```python
from build123d import *

# Parameters (mm, degrees)
SKETCH_1_R               = 15
SKETCH_1_R_2             = 1.25
EXTRUDE_2_DEPTH          = 5
SKETCH_3_R               = 5
EXTRUDE_4_DEPTH          = 1
SKETCH_4_R               = 3
CUT_EXTRUDE_1_DEPTH      = 5.5
CUT_EXTRUDE_2_DEPTH      = 78
CUT_EXTRUDE_2_DEPTH_BACK = 5.5
SKETCH_5_R               = 1.5


with BuildPart() as part:
    # ｽｹｯﾁ1 → ﾎﾞｽ - 押し出し2 (new body)
    with BuildSketch(Plane(origin=(0, 0, 0), x_dir=(0, 0, -1), z_dir=(1, 0, 0))):
        with Locations((27.213776389, 17.709467549)):
            Circle(SKETCH_1_R)
        with Locations((27.213776389, 29.709467549)):
            Circle(SKETCH_1_R_2, mode=Mode.SUBTRACT)
        with Locations((35.699057763, 26.194748924)):
            Circle(SKETCH_1_R_2, mode=Mode.SUBTRACT)
        with Locations((18.728495014, 26.194748924)):
            Circle(SKETCH_1_R_2, mode=Mode.SUBTRACT)
        with Locations((15.213776389, 17.709467549)):
            Circle(SKETCH_1_R_2, mode=Mode.SUBTRACT)
        with Locations((35.699057763, 9.224186175)):
            Circle(SKETCH_1_R_2, mode=Mode.SUBTRACT)
        with Locations((39.213776389, 17.709467549)):
            Circle(SKETCH_1_R_2, mode=Mode.SUBTRACT)
        with Locations((18.728495014, 9.224186175)):
            Circle(SKETCH_1_R_2, mode=Mode.SUBTRACT)
        with Locations((27.213776389, 5.709467549)):
            Circle(SKETCH_1_R_2, mode=Mode.SUBTRACT)
    extrude(amount=EXTRUDE_2_DEPTH)

    # ｽｹｯﾁ3 → ﾎﾞｽ - 押し出し4 (add)
    with BuildSketch(Plane(origin=(0, 0, 0), x_dir=(0, 0, -1), z_dir=(1, 0, 0))):
        with Locations((27.213776389, 17.709467549)):
            Circle(SKETCH_3_R)
    extrude(amount=-EXTRUDE_4_DEPTH)

    # ｽｹｯﾁ4 → ｶｯﾄ - 押し出し1 (cut)
    with BuildSketch(Plane(origin=(5, 0, 0), x_dir=(0, 0, -1), z_dir=(1, 0, 0))):
        with Locations((27.213776389, 17.709467549)):
            Circle(SKETCH_4_R)
    extrude(amount=-CUT_EXTRUDE_1_DEPTH, mode=Mode.SUBTRACT)

    # ｽｹｯﾁ5 → ｶｯﾄ - 押し出し2 (cut, two sides: drawn at the far end of the back side and taken through both)
    with BuildSketch(Plane.ZY.offset(-CUT_EXTRUDE_2_DEPTH_BACK)):
        with Locations(Location((-27.213776389, 17.709467549, 0), (0, 0, 180))):
            Circle(SKETCH_5_R)
    extrude(amount=CUT_EXTRUDE_2_DEPTH + CUT_EXTRUDE_2_DEPTH_BACK, mode=Mode.SUBTRACT)


solid = part.part
```
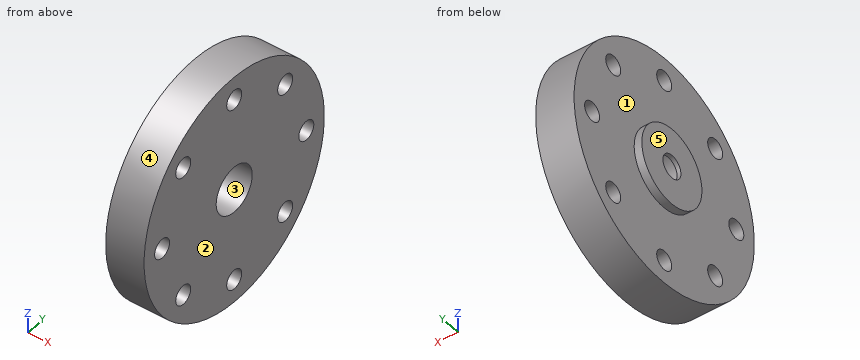
Could you check a few things on this model? Use its own coordinates, in mm. Face numbers are marked on the shaded views. A direction names the side the tool comes from. Round coordinates to 2 decimals unless told otherwise and drop trailing zeros. Loops run counter-clockwise (first coordinate to the right, second up) from the corner with the lowest first, then second, coordinate; pieces in that order, holes last. Notation, with made-up numbers: (44, -29.75) - (61, -29.75) arc R27 ccw to (61, -12.75) - close; hole circle Ø1 at (-30, 45.25). An arc over 180 degrees is marked (long way). Answer in a Markdown table with one row per item. Add a question column.
(1) I need wall thicknesses on line 1 along Y through (x, z) = (2.95, -19); line 2 along Y through (x, z) = (3.3, -27.5); line 3 along X through (y, z) = (10, -34). Which ranges of each line are inside material? Lowest first, please.
(2) If we section it at A-A (z = -18.5): Please give me the cut outline in (x, y).
(3) If we mould it in two halves opening along Y, with no side actions, what happens to the marked faces 3, 4 and 5? For each: pulls with the +Y half, pulls with the -Y half, needs draft (parallel to the pull), parting line crosses it, or undercut.
(4) If we section it at B-B (y = 27): Please give me the cut outline in (x, z), plus the area to 3 significant figures.
(5) If we section it at C-C (z = -28): Please give me the cut outline in (x, y).
(6) If we section it at D-D (y = 30.5): Please give me the cut outline in (x, z).
(7) I'm going to push flat-ended pins straight in: pin 1 (1 mm diameter, centred on x = 1.5, z = -18.5, fed in from +Y); pin 2 (2 mm diameter, centred on x = 2.5, z = -29.5, fed in from +Y); pin 3 (5 mm diameter, centred on y = 9.5, z = -23, fed in from -X). Where does each tip first touch, or does it pass through?
(8) For the marked faces 1 and 2, which set-ups out of +Z, -Z, +X, -X, +Y, -Y let a thin tool reach every point of the face, with its end or its side?
Model answer:
| question | item | result |
|---|---|---|
| 1 | line 1 | y = 5.16 to 8, 10.44 to 24.97, 27.41 to 30.26 |
| 1 | line 2 | y = 2.71 to 4.49, 6.93 to 14.72, 20.7 to 28.49, 30.93 to 32.71 |
| 1 | line 3 | x = 0 to 5 |
| 2 | outline | (0, 5.5) - (5, 5.5) - (5, 8) - (0, 8) - close; (0, 10.45) - (5, 10.45) - (5, 24.97) - (0, 24.97) - close; (0, 27.42) - (5, 27.42) - (5, 29.92) - (0, 29.92) - close |
| 3 | face 3 | undercut |
| 3 | face 4 | parting line crosses it |
| 3 | face 5 | needs draft |
| 4 | outline | (0, -38.99) - (5, -38.99) - (5, -36.66) - (0, -36.66) - close; (0, -34.74) - (5, -34.74) - (5, -19.68) - (0, -19.68) - close; (0, -17.77) - (5, -17.77) - (5, -15.44) - (0, -15.44) - close |
| 4 | area | 98.6 mm² |
| 5 | outline | (-1, 12.77) - (0, 12.77) - (0, 6.68) - (5, 6.68) - (5, 14.81) - (-0.5, 14.81) - (-0.5, 16.43) - (-1, 16.43) - close; (-1, 18.99) - (-0.5, 18.99) - (-0.5, 20.6) - (5, 20.6) - (5, 28.74) - (0, 28.74) - (0, 22.65) - (-1, 22.65) - close; (0, 2.73) - (5, 2.73) - (5, 4.74) - (0, 4.74) - close; (0, 30.68) - (5, 30.68) - (5, 32.69) - (0, 32.69) - close |
| 6 | outline | (0, -35.05) - (5, -35.05) - (5, -28.18) - (0, -28.18) - close; (0, -26.25) - (5, -26.25) - (5, -19.38) - (0, -19.38) - close |
| 7 | pin 1 | stops at y = 30.26 |
| 7 | pin 2 | stops at y = 32.65 |
| 7 | pin 3 | stops at x = 0 |
| 8 | face 1 | -X |
| 8 | face 2 | +Z, -Z, +X, +Y, -Y |
